Geometry: final body of the model. Coordinates: model frame, mm. A direction names the side the tool comes from. Give positions to 0.01 mm unless a question says otherwise; leave off trailing zeros. Loops run counter-clockwise (first coordinate to the right, second up) from the corner with the lowest first, then second, coordinate; pieces in that order, holes last. Notation, with made-up numbers: M 3.25,37 L 18.25,37 A19 ccw 18.25,41 Z; hole C 78,47.25 d8. An arc over 180 degrees is marked long. Put each result on its own line as item: value.
```python
from build123d import *

# Parameters (mm, degrees)
SKETCH_R     = 51
PAD_DEPTH    = 60
THICKNESS_T  = 1.4
SKETCH001_R  = 23.5
PAD001_DEPTH = 60


with BuildPart() as part:
    # Sketch → Pad (new body)
    with BuildSketch(Plane.XY):
        Circle(SKETCH_R)
    extrude(amount=PAD_DEPTH)

    # Thickness
    thickness_openings = [part.faces().sort_by_distance(p)[0] for p in [
        (0, 0, 60),
    ]]
    offset(amount=THICKNESS_T, openings=thickness_openings, kind=Kind.INTERSECTION)

    # Sketch001 (on Face2 of Thickness) → Pad001 (join)
    with BuildSketch(Plane.XY):
        Circle(SKETCH001_R)
    extrude(amount=PAD001_DEPTH)


solid = part.part
```
Item 1: Mould query, pull axis X, two halves, no side actions, for faces 3 (the cylindrical face through (-11.056, -49.787, 29.58)), 4 (the cylindrical face through (-6.821, 51.954, 28.87)), 5 (the flat face through (-1, 1, -1.4)). Classes: pulls with the +X half, pulls with the -X half, needs draft (parallel to the pull), parting line crosses it, or undercut.
Output values:
face 3: undercut
face 4: parting line crosses it
face 5: needs draft
Item 2: Section B-B on y = 0. Output: boundary loops of the cut face in (x, z).
Output values:
outline: M -52.4,-1.4 L 52.4,-1.4 L 52.4,60 L 51,60 L 51,0 L 23.5,0 L 23.5,60 L -23.5,60 L -23.5,0 L -51,0 L -51,60 L -52.4,60 Z
Item 3: Section D-D on y = -35. Output: boundary loops of the cut face in (x, z).
Output values:
outline: M -39,-1.4 L 39,-1.4 L 39,60 L 37.09,60 L 37.09,0 L -37.09,0 L -37.09,60 L -39,60 Z
Item 4: Section A-A on z = 31. Output: boundary loops of the cut face in (x, y).
Output values:
outline: C 0,0 d104.8; C 0,0 d47; hole C 0,0 d102
Item 5: Pin query (flat end, axial travel): pin 1 Ø1 at (x, y) = (39.5, 27) entering from +Z; pin 2 Ø3 at (y, z) = (-14.5, 21.5) entering from +X; pin 3 Ø4 at (y, z) = (-37, 36.5) entering from -X. Return the tip coordinate at first contact, or that it passes through.
Output values:
pin 1: z = 0
pin 2: x = 50.76
pin 3: x = -39
Item 6: Line query: probe 1 along Y at (x, z) = (0, 33); probe 2 along Y at (x, z) = (15.5, 49.5); probe 3 along X at (y, z) = (21.5, 53.5). Output: solid intervals per line, ascending. Write a range as [from, to].
Output values:
probe 1: [-52.4, -51], [-23.5, 23.5], [51, 52.4]
probe 2: [-50.06, -48.59], [-17.66, 17.66], [48.59, 50.06]
probe 3: [-47.79, -46.25], [-9.49, 9.49], [46.25, 47.79]
Item 7: Set-up query: faces 1 (the flat face through (0, 0, 60)), 2 (the flat face through (22, -11, 0)). Return all of +Z, -Z, +X, -X, +Y, -Y with unobstructed straight access to the full face (end or side cutting, diameter ignored); none if empty.
Output values:
face 1: +Z, +X, -X, +Y, -Y
face 2: +Z
